from build123d import *

# Parameters (mm, degrees)
SKETCH_1_W          = 100
SKETCH_1_H          = 30
EXTRUDE_1_DEPTH     = 50
SKETCH_2_W          = 22
SKETCH_2_H          = 42
CUT_EXTRUDE_1_DEPTH = 113.805141727
SKETCH_3_R          = 2.1
CUT_EXTRUDE_3_DEPTH = 20
SKETCH_4_R          = 1.6
CUT_EXTRUDE_4_DEPTH = 20


with BuildPart() as part:
    # 草图1 → 凸台-拉伸1 (new body)
    with BuildSketch(Plane(origin=(0, 0, 0), x_dir=(1, 0, 0), z_dir=(0, 1, 0))):
        Rectangle(SKETCH_1_W, SKETCH_1_H)
    extrude(amount=EXTRUDE_1_DEPTH)

    # 草图2 → 切除-拉伸1 (cut, through all)
    with BuildSketch(Plane.ZY.offset(50)):
        with Locations((0, 25)):
            Rectangle(SKETCH_2_W, SKETCH_2_H)
    extrude(amount=-CUT_EXTRUDE_1_DEPTH, mode=Mode.SUBTRACT)

    # 草图3 → 切除-拉伸3 (cut)
    with BuildSketch(Plane.XZ):
        with Locations(Location((13, 8, 0), (0, 0, 270))):
            Circle(SKETCH_3_R)
        with Locations(Location((-13, 8, 0), (0, 0, 270))):
            Circle(SKETCH_3_R)
    extrude(amount=-CUT_EXTRUDE_3_DEPTH, mode=Mode.SUBTRACT)

    # 草图4 → 切除-拉伸4 (cut)
    with BuildSketch(Plane(origin=(0, 50, 0), x_dir=(1, 0, 0), z_dir=(0, 1, 0))):
        with Locations(Location((-42, 7, 0), (0, 0, 270))):
            Circle(SKETCH_4_R)
        with Locations(Location((-42, -7, 0), (0, 0, 270))):
            Circle(SKETCH_4_R)
        with Locations(Location((42, 7, 0), (0, 0, 270))):
            Circle(SKETCH_4_R)
        with Locations(Location((42, -7, 0), (0, 0, 270))):
            Circle(SKETCH_4_R)
    extrude(amount=-CUT_EXTRUDE_4_DEPTH, mode=Mode.SUBTRACT)


solid = part.part
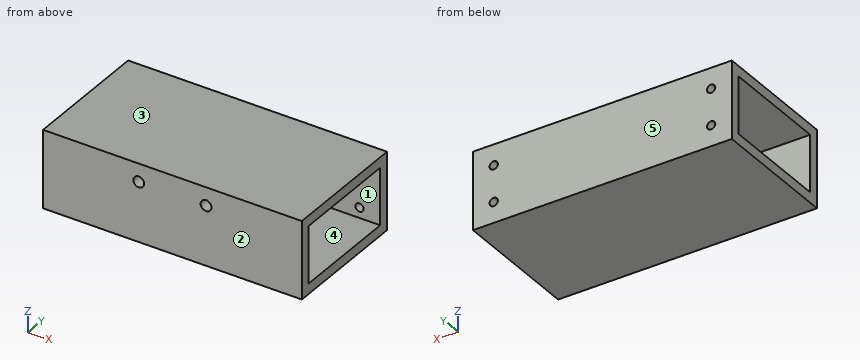
Could you check a few things on this model? Use its own coordinates, in mm. Face numbers are marked on the shaded views. A direction names the side the tool comes from. Coordinates: 2 decimals unless noted, no trailing zeros. Loops run counter-clockwise (first coordinate to the right, second up) from the corner with the lowest first, then second, coordinate; pieces in that order, holes last. Notation, with made-up numbers: (-11.5, 0) -> (-2.5, 0) arc R31 ccw to (-2.5, 36) -> close; hole circle Ø8 at (87, 26.25). An arc over 180 degrees is marked (long way). Answer in a Markdown table with one row per item.
(1) Thinking about a two-plate mould opening in Z: for the marked faces 1, 2 and 3, which applies, released by +Z, released by -Z, zero draft, split by the parting line, or undercut?
Results found:
| item | result |
|---|---|
| face 1 | undercut |
| face 2 | zero draft |
| face 3 | released by +Z |
(2) Imagine slicing it at B-B (z = -0.25). List the corners of the cut face in (x, y) for me, plus the area to 3 significant figures.
Results found:
| item | result |
|---|---|
| outline | (-50, 0) -> (50, 0) -> (50, 4) -> (-50, 4) -> close; (-50, 46) -> (50, 46) -> (50, 50) -> (-50, 50) -> close |
| area | 800 mm^2 |
(3) Imagine slicing it at D-D (x = -13). List the corners of the cut face in (y, z) for me, plus the area to 3 significant figures.
Results found:
| item | result |
|---|---|
| outline | (0, -15) -> (50, -15) -> (50, 15) -> (0, 15) -> (0, 10.1) -> (4, 10.1) -> (4, 11) -> (46, 11) -> (46, -11) -> (4, -11) -> (4, 5.9) -> (0, 5.9) -> close |
| area | 559 mm^2 |
(4) Imagine slicing it at A-A (x = -42). List the corners of the cut face in (y, z) for me, plus the area to 3 significant figures.
Results found:
| item | result |
|---|---|
| outline | (0, -15) -> (50, -15) -> (50, -8.6) -> (46, -8.6) -> (46, -11) -> (4, -11) -> (4, 11) -> (46, 11) -> (46, 8.6) -> (50, 8.6) -> (50, 15) -> (0, 15) -> close; (46, -5.4) -> (50, -5.4) -> (50, 5.4) -> (46, 5.4) -> close |
| area | 550 mm^2 |
(5) If I drill on probe 1 along X at (y, z) = (0.8, 8); probe 2 along X at (y, z) = (48.15, 7); probe 3 along Y at (x, z) = (-27, 0.5), over which ranges is the centre line in solid material (lowest first)?
Results found:
| item | result |
|---|---|
| probe 1 | x = -50 to -15.1, -10.9 to 10.9, 15.1 to 50 |
| probe 2 | x = -50 to -43.6, -40.4 to 40.4, 43.6 to 50 |
| probe 3 | y = 0 to 4, 46 to 50 |
(6) Imagine slicing it at C-C (y = 34). List the corners of the cut face in (x, z) for me.
Results found:
| item | result |
|---|---|
| outline | (-50, -15) -> (50, -15) -> (50, -11) -> (-50, -11) -> close; (-50, 11) -> (50, 11) -> (50, 15) -> (-50, 15) -> close |
(7) For the marked faces 4 and 5, which set-ups out of +Z, -Z, +X, -X, +Y, -Y let a thin tool reach every point of the face, with its end or its side?
Results found:
| item | result |
|---|---|
| face 4 | +X, -X |
| face 5 | +Z, -Z, +X, -X, +Y |
